from build123d import *

# Parameters (mm, degrees)
SKETCH1_W           = 53
SKETCH1_H           = 98
BOSS_EXTRUDE1_DEPTH = 80
SKETCH2_W           = 90
SKETCH2_H           = 76
CUT_EXTRUDE1_DEPTH  = 49
SKETCH3_W           = 51
SKETCH3_H           = 2
CUT_EXTRUDE2_DEPTH  = 5
SKETCH5_W           = 2
SKETCH5_H           = 76
CUT_EXTRUDE3_DEPTH  = 5
CUT_EXTRUDE4_DEPTH  = 1.8
SKETCH8_R           = 1.3
BOSS_EXTRUDE3_DEPTH = 2.5
FILLET2_R           = 1.5
SKETCH9_R           = 1.3
BOSS_EXTRUDE4_DEPTH = 2.5
FILLET4_R           = 1.5
CUT_EXTRUDE6_REACH  = 53.2
SKETCH14_W          = 64.2
SKETCH14_H          = 43.4
SKETCH15_W          = 74.2
SKETCH15_H          = 53.4
CUT_EXTRUDE7_DEPTH  = 2
CUT_EXTRUDE8_REACH  = 51.2
SKETCH16_R          = 1.3
CUT_EXTRUDE12_REACH = 106
SKETCH29_R          = 1.65


with BuildPart() as part:
    # Sketch1 → Boss-Extrude1 (new body)
    with BuildSketch(Plane(origin=(0, 0, 0), x_dir=(1, 0, 0), z_dir=(0, 1, 0))):
        Rectangle(SKETCH1_W, SKETCH1_H)
    extrude(amount=BOSS_EXTRUDE1_DEPTH)

    # Sketch2 → Cut-Extrude1 (cut)
    with BuildSketch(Plane(origin=(26.5, 0, 0), x_dir=(0, 0, -1), z_dir=(1, 0, 0))):
        with Locations((0, 42)):
            Rectangle(SKETCH2_W, SKETCH2_H)
    extrude(amount=-CUT_EXTRUDE1_DEPTH, mode=Mode.SUBTRACT)

    # Sketch3 → Cut-Extrude2 (cut)
    with BuildSketch(Plane(origin=(0, 80, 0), x_dir=(1, 0, 0), z_dir=(0, 1, 0))):
        Polygon((-26.5, -49), (26.5, -49), (26.5, -47), (-24.5, -47), (-26.5, -47), align=None)
        Polygon((-26.5, 49), (-26.5, -47), (-24.5, -47), (-24.5, 47), (-24.5, 49), align=None)
        with Locations((1, 48)):
            Rectangle(SKETCH3_W, SKETCH3_H)
    extrude(amount=-CUT_EXTRUDE2_DEPTH, mode=Mode.SUBTRACT)

    # Sketch5 → Cut-Extrude3 (cut)
    with BuildSketch(Plane(origin=(26.5, 0, 0), x_dir=(0, 0, -1), z_dir=(1, 0, 0))):
        with Locations((-46, 42)):
            Rectangle(SKETCH5_W, SKETCH5_H)
        Polygon((-45, 4), (-47, 4), (-47, 2), (47, 2), (47, 4), (45, 4), align=None)
        with Locations((46, 42)):
            Rectangle(SKETCH5_W, SKETCH5_H)
    extrude(amount=-CUT_EXTRUDE3_DEPTH, mode=Mode.SUBTRACT)

    # Sketch6 → Cut-Extrude4 (cut)
    with BuildSketch(Plane(origin=(26.5, 0, 0), x_dir=(0, 0, -1), z_dir=(1, 0, 0))):
        Polygon((47, 75), (47, 2), (-47, 2), (-47, 75), (-49, 75), (-49, 0), (49, 0), (49, 75), align=None)
    extrude(amount=-CUT_EXTRUDE4_DEPTH, mode=Mode.SUBTRACT)

    # Sketch8 → Boss-Extrude3 (add)
    with BuildSketch(Plane(origin=(24.7, 0, 0), x_dir=(0, 0, -1), z_dir=(1, 0, 0))):
        with BuildLine():
            Line((-49, 10), (-51, 10))
            ThreePointArc((-51, 10), (-55, 14), (-51, 18))
            Line((-51, 18), (-49, 18))
            Line((-49, 18), (-49, 10))
        make_face()
        with Locations((-52.4, 14)):
            Circle(SKETCH8_R, mode=Mode.SUBTRACT)
        with BuildLine():
            Line((-49, 65), (-49, 57))
            Line((-49, 57), (-51, 57))
            ThreePointArc((-51, 57), (-55, 61), (-51, 65))
            Line((-51, 65), (-49, 65))
        make_face()
        with Locations((-52.4, 61)):
            Circle(SKETCH8_R, mode=Mode.SUBTRACT)
        with BuildLine():
            Line((49, 10), (49, 18))
            Line((49, 18), (51, 18))
            ThreePointArc((51, 18), (55, 14), (51, 10))
            Line((51, 10), (49, 10))
        make_face()
        with Locations((52.4, 14)):
            Circle(SKETCH8_R, mode=Mode.SUBTRACT)
        with BuildLine():
            Line((49, 65), (51, 65))
            ThreePointArc((51, 65), (55, 61), (51, 57))
            Line((51, 57), (49, 57))
            Line((49, 57), (49, 65))
        make_face()
        with Locations((52.4, 61)):
            Circle(SKETCH8_R, mode=Mode.SUBTRACT)
    extrude(amount=-BOSS_EXTRUDE3_DEPTH)

    # Fillet2
    fillet2_edges = [part.edges().sort_by_distance(p)[0] for p in [
        (22.2, 14, 49),
        (23.45, 18, 49),
        (23.45, 10, 49),
        (22.2, 61, 49),
        (23.45, 65, 49),
        (23.45, 57, 49),
        (22.2, 14, -49),
        (23.45, 10, -49),
        (23.45, 18, -49),
        (22.2, 61, -49),
        (23.45, 57, -49),
        (23.45, 65, -49),
    ]]
    fillet(fillet2_edges, radius=FILLET2_R)

    # Sketch9 → Boss-Extrude4 (add)
    with BuildSketch(Plane(origin=(0, 75, 0), x_dir=(1, 0, 0), z_dir=(0, 1, 0))):
        with BuildLine():
            Line((-26.5, 4), (-28.5, 4))
            ThreePointArc((-28.5, 4), (-32.5, 0), (-28.5, -4))
            Line((-28.5, -4), (-26.5, -4))
            Line((-26.5, -4), (-26.5, 4))
        make_face()
        with Locations((-29.9, 0)):
            Circle(SKETCH9_R, mode=Mode.SUBTRACT)
    extrude(amount=-BOSS_EXTRUDE4_DEPTH)

    # Fillet4
    fillet4_edges = [part.edges().sort_by_distance(p)[0] for p in [
        (-26.5, 72.5, 0),
        (-26.5, 73.75, -4),
        (-26.5, 73.75, 4),
    ]]
    fillet(fillet4_edges, radius=FILLET4_R)

    # Sketch14 → Cut-Extrude6 (cut, up to next)
    with BuildSketch(Plane.ZY.offset(26.5), mode=Mode.PRIVATE) as cut_extrude6_sk1:
        with Locations((0, 33.7)):
            Rectangle(SKETCH14_W, SKETCH14_H)
    cut_extrude6_tool1 = extrude(cut_extrude6_sk1.sketch, amount=-CUT_EXTRUDE6_REACH, mode=Mode.PRIVATE) & part.part
    add(cut_extrude6_tool1.solids().sort_by_distance((-26.5, 33.7, 0))[0], mode=Mode.SUBTRACT)

    # Sketch15 → Cut-Extrude7 (cut)
    with BuildSketch(Plane.ZY.offset(26.5)):
        with Locations((0, 33.7)):
            Rectangle(SKETCH15_W, SKETCH15_H)
    extrude(amount=-CUT_EXTRUDE7_DEPTH, mode=Mode.SUBTRACT)

    # Sketch16 → Cut-Extrude8 (cut, up to next)
    with BuildSketch(Plane.ZY.offset(24.5), mode=Mode.PRIVATE) as cut_extrude8_sk1:
        with Locations((0, 57.9)):
            Circle(SKETCH16_R)
    cut_extrude8_tool1 = extrude(cut_extrude8_sk1.sketch, amount=-CUT_EXTRUDE8_REACH, mode=Mode.PRIVATE) & part.part
    add(cut_extrude8_tool1.solids().sort_by_distance((-24.5, 57.9, 0))[0], mode=Mode.SUBTRACT)
    # Sketch16 → Cut-Extrude8 (cut, up to next)
    with BuildSketch(Plane.ZY.offset(24.5), mode=Mode.PRIVATE) as cut_extrude8_sk2:
        with Locations((0, 9.5)):
            Circle(SKETCH16_R)
    cut_extrude8_tool2 = extrude(cut_extrude8_sk2.sketch, amount=-CUT_EXTRUDE8_REACH, mode=Mode.PRIVATE) & part.part
    add(cut_extrude8_tool2.solids().sort_by_distance((-24.5, 9.5, 0))[0], mode=Mode.SUBTRACT)

    # Sketch29 → Cut-Extrude12 (cut, up to next)
    with BuildSketch(Plane(origin=(0, 0, -49), x_dir=(-1, 0, 0), z_dir=(0, 0, -1)), mode=Mode.PRIVATE) as cut_extrude12_sk1:
        with Locations((14.5, 20)):
            Circle(SKETCH29_R)
    cut_extrude12_tool1 = extrude(cut_extrude12_sk1.sketch, amount=-CUT_EXTRUDE12_REACH, mode=Mode.PRIVATE) & part.part
    add(cut_extrude12_tool1.solids().sort_by_distance((-14.5, 20, -49))[0], mode=Mode.SUBTRACT)


solid = part.part
Input: part model. Units: mm. Frame: model coordinates. A direction names the side the tool comes from. Round coordinates to 2 decimals unless told otherwise and drop trailing zeros. Order: outer loops, then holes, each group sorted by start corner. A loop starts at its lowest first (then second) coordinate and runs counter-clockwise, first axis right, second up. Notation, with made-up numbers: (45.5, 89.5) - (101.5, 89.5) arc R30 ccw to (101.5, 113.5) - close; hole circle Ø4 at (61, -23.75). An arc over 180 degrees is marked (long way). Answer as a JSON object with one key per item and string values. Group by question number.
(1) Pin query (flat end, axial travel): P1, Ø4, axis at y = 57.9, z = 0, coming from the -X side; P2, Ø1.3, axis at x = -30, z = -1.5, coming from the -Y side; P3, Ø1.5, axis at y = 44, z = -30.5, coming from the +X side; P4, Ø2, axis at y = 14, z = 52, coming from the -X side. Return the tip coordinate at first contact, or that it passes through.
(2) Draft query along Y for faces 1 (the face through (0, 4, 1)), 2 (the face through (23, 38, -47)), 3 (the face through (-23.514, 56.747, 0.6)). Return one class per face: released by +Y, released by -Y, zero draft, split by the parting line, or undercut.
(3) Material intervals for probe 1 along Z at (x, y) = (20.5, 9); probe 2 along Y at (x, z) = (23, 52); probe 3 along Y at (x, z) = (-4.5, 7), sorted ascending. Write a range as from..to.
(4) Cut plane C-C (y = 14). Count the separate pieces of the cut face and the enclosed holes in it, then the cut area to 3 significant figures.
(5) Cut plane B-B (x = -14.5). Return loops of the section in (y, z).
(6) Cut plane A-A (z = -22.5). Return loops of the section in (x, y).
(7) Cut plane D-D (y = 30). Return loops of the section in (x, z).
(8) Reachability of faces 4 (the face through (0, 41, -45)), 5 (the face through (-28.78, 72.5, -0.94)), 6 (the face through (-24.5, 10, -9)) from +Z, -Z, +X, -X, +Y, -Y: full face, straight path, thin tool, end or side. Return the list, or none.
Here are the results:
{
 "1": {"P1": "stops at x = -24.5", "P2": "stops at y = 72.5", "P3": "passes through", "P4": "stops at x = 22.2"},
 "2": {"face 1": "released by +Y", "face 2": "zero draft", "face 3": "undercut"},
 "3": {"probe 1": "z = -49..-45, 45..49", "probe 2": "y = 10.13..12.76, 15.24..17.87, 57.13..59.76, 62.24..64.87", "probe 3": "y = 0..4"},
 "4": {"separate pieces": "4", "enclosed holes": "0", "area": "498 mm^2"},
 "5": {"outline": "(0, -49) - (18.35, -49) - (18.35, -45) - (4, -45) - (4, 45) - (80, 45) - (80, 47) - (75, 47) - (75, 49) - (0, 49) - close; (21.65, -49) - (75, -49) - (75, -47) - (80, -47) - (80, -45) - (21.65, -45) - close"},
 "6": {"outline": "(-26.5, 0) - (24.7, 0) - (24.7, 2) - (21.5, 2) - (21.5, 4) - (-22.5, 4) - (-22.5, 12) - (-24.5, 12) - (-24.5, 7) - (-26.5, 7) - close; (-26.5, 60.4) - (-24.5, 60.4) - (-24.5, 55.4) - (-22.5, 55.4) - (-22.5, 80) - (-24.5, 80) - (-24.5, 75) - (-26.5, 75) - close"},
 "7": {"outline": "(-26.5, -49) - (24.7, -49) - (24.7, -47) - (21.5, -47) - (21.5, -45) - (-22.5, -45) - (-22.5, -32.1) - (-24.5, -32.1) - (-24.5, -37.1) - (-26.5, -37.1) - close; (-26.5, 37.1) - (-24.5, 37.1) - (-24.5, 32.1) - (-22.5, 32.1) - (-22.5, 45) - (21.5, 45) - (21.5, 47) - (24.7, 47) - (24.7, 49) - (-26.5, 49) - close"},
 "8": {"face 4": "+X, +Y", "face 5": "+Z, -Z, -X, -Y", "face 6": "-X"}
}
